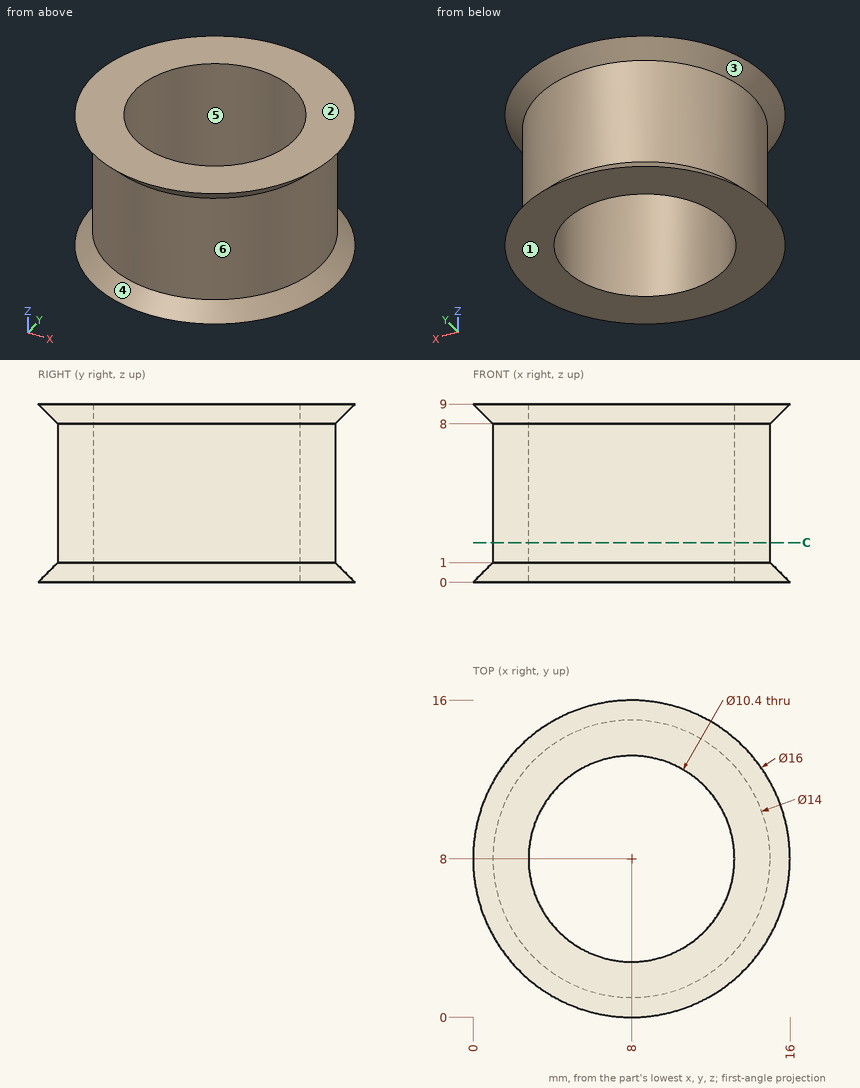
Print and shaded views of the part. All mm, measured from the part's lowest x, y and z. A direction names the side the tool comes from. Round coordinates to 2 decimals unless told otherwise and drop trailing zeros. Write each loop counter-clockwise with the first axis right and the second up, starting at its lowest first coordinate (ties: lowest second). Pieces come first, ordered by that corner, then holes. Notation, with made-up numbers: (-14.75, 19.5) -> (22.25, 19.5) arc R12 ccw to (22.25, 26.5) -> close; hole circle Ø3 at (50.25, 48). An arc over 180 degrees is marked (long way). Answer in a Markdown table with one row per item. Add a question column.
Item 1: Mould opens along Z. For the marked faces 1, 2, 3 and 4 say: pulls with the +Z half, pulls with the -Z half, needs draft (parallel to the pull), parting line crosses it, or undercut.
Item 2: Drop flat-ended pins along their axis: pin 1 Ø1.5 at (x, y) = (4, 2.5) entering from -Z; pin 2 Ø2 at (x, z) = (13.5, 3) entering from -Y; pin 3 Ø4 at (y, z) = (2, 3) entering from -X; pin 4 Ø2 at (x, z) = (9, 1.5) entering from +Y. Give the stop position or say it passes through.
Item 3: Which spindle directions (+Z, -Z, +X, -X, +Y, -Y) get a long thin tool onto all of the face, cutting with end or side? Do the marked faces 5 and 6. Say none if no direction does.
Item 4: Drill centre lines: line 1 (Y direction, x = 8, z = 7.25); line 2 (Z direction, x = 0.5, y = 6.25); line 3 (Y direction, x = 4.25, z = 7.5). Where is each one in solid material? Low to high. Write a range as from..to.
Item 5: Saw through at C-C, the plane z = 2. Write the cut outline in (x, y), then the cut area to 3 significant figures.
Findings below:
| question | item | result |
|---|---|---|
| 1 | face 1 | pulls with the -Z half |
| 1 | face 2 | pulls with the +Z half |
| 1 | face 3 | undercut |
| 1 | face 4 | undercut |
| 2 | pin 1 | stops at z = 0 |
| 2 | pin 2 | stops at y = 2.64 |
| 2 | pin 3 | stops at x = 2.26 |
| 2 | pin 4 | stops at y = 15.44 |
| 3 | face 5 | +Z, -Z |
| 3 | face 6 | none |
| 4 | line 1 | y = 1..2.8, 13.2..15 |
| 4 | line 2 | z = 0..0.3, 8.7..9 |
| 4 | line 3 | y = 2.09..4.4, 11.6..13.91 |
| 5 | outline | circle Ø14 at (8, 8); hole circle Ø10.4 at (8, 8) |
| 5 | area | 69.0 mm^2 |
